Geometry: see drawing. Coordinates: mm, zero at the bounding-box minimum. A direction names the side the tool comes from. Round coordinates to 2 decimals unless told otherwise and drop trailing zeros. Loops run counter-clockwise (first coordinate to the right, second up) from the corner with the lowest first, then second, coordinate; pieces in that order, holes last.
(1) Material intervals for probe 1 along Y at (x, z) = (38, 1.5); probe 2 along X at (y, z) = (9, 1.25); probe 3 along Z at (x, y) = (33.5, 70.5), sorted ascending.
(2) Set-up query: the marked faces 1, 2 and 3. Return all of +Z, -Z, +X, -X, +Y, -Y with unobstructed straight access to the full face (end or side cutting, diameter ignored); none if empty.
(3) Section A-A, the plane x = 22.5. Return the cut outline in (y, z), plus the area to 3 significant figures.
(4) Section C-C, the plane z = 8. Return the cut outline in (x, y), plus the area to 3 significant figures.
(5) First-contact query: pin 1 Ø7 at (y, z) = (4.5, 3.5) entering from +X; pin 2 Ø1.9 at (x, y) = (45, 44) entering from +Z; pin 3 Ø5 at (x, z) = (39, 10) entering from +Y; pin 4 Ø6 at (x, y) = (11, 51) entering from -Z. Flat tips, straight axial feed; report the tip coordinate or a pass-through.
(6) Section B-B, the plane y = 36.5. Return the cut outline in (x, z), plus the area to 3 significant figures.
(7) Section D-D, the plane z = 3.75. Return the cut outline in (x, y), plus the area to 3 significant figures.
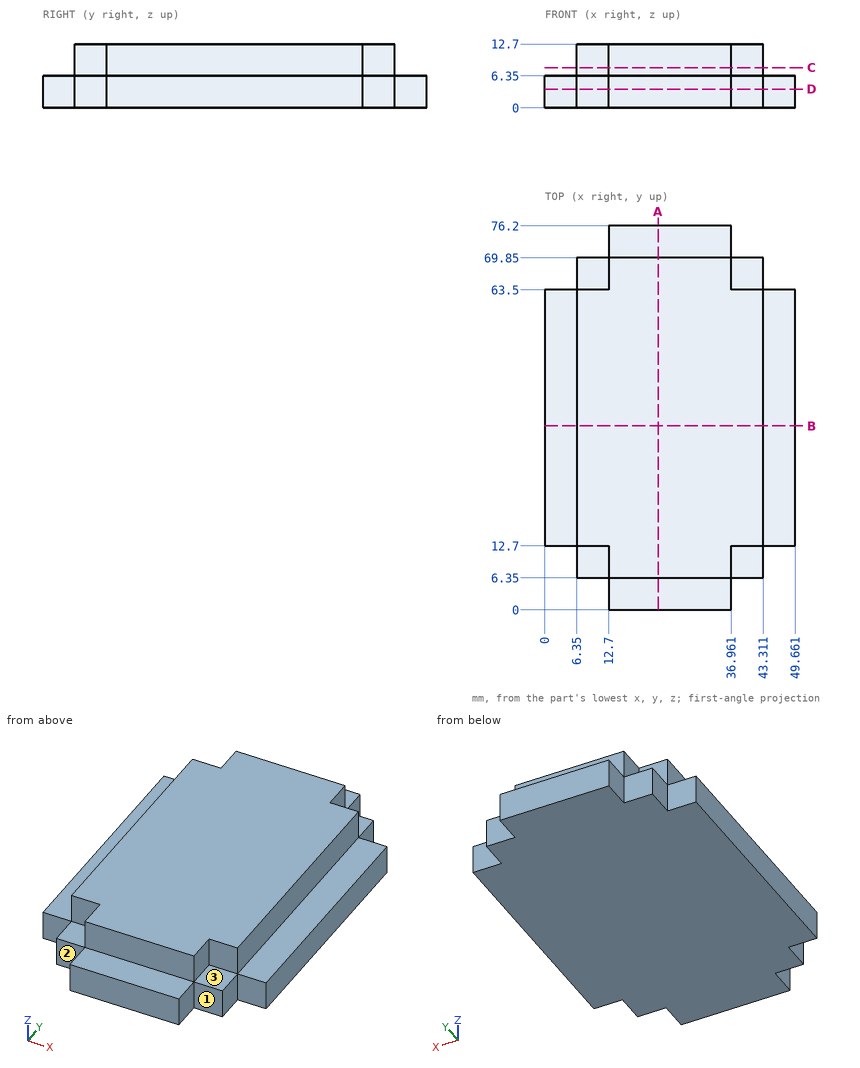
Output values:
1. probe 1: y = 6.35 to 69.85
1. probe 2: x = 6.35 to 43.31
1. probe 3: z = 0 to 6.35
2. face 1: +Z, -Z, +X, -Y
2. face 2: +Z, -Z, -X, -Y
2. face 3: +Z, +X, -Y
3. outline: (0, 0) - (76.2, 0) - (76.2, 6.35) - (69.85, 6.35) - (69.85, 12.7) - (6.35, 12.7) - (6.35, 6.35) - (0, 6.35) - close
3. area: 887 mm2
4. outline: (6.35, 12.7) - (12.7, 12.7) - (12.7, 6.35) - (36.96, 6.35) - (36.96, 12.7) - (43.31, 12.7) - (43.31, 63.5) - (36.96, 63.5) - (36.96, 69.85) - (12.7, 69.85) - (12.7, 63.5) - (6.35, 63.5) - close
4. area: 2,190 mm2
5. pin 1: stops at x = 43.31
5. pin 2: stops at z = 6.35
5. pin 3: stops at y = 69.85
5. pin 4: stops at z = 0
6. outline: (0, 0) - (49.66, 0) - (49.66, 6.35) - (43.31, 6.35) - (43.31, 12.7) - (6.35, 12.7) - (6.35, 6.35) - (0, 6.35) - close
6. area: 550 mm2
7. outline: (0, 12.7) - (6.35, 12.7) - (6.35, 6.35) - (12.7, 6.35) - (12.7, 0) - (36.96, 0) - (36.96, 6.35) - (43.31, 6.35) - (43.31, 12.7) - (49.66, 12.7) - (49.66, 63.5) - (43.31, 63.5) - (43.31, 69.85) - (36.96, 69.85) - (36.96, 76.2) - (12.7, 76.2) - (12.7, 69.85) - (6.35, 69.85) - (6.35, 63.5) - (0, 63.5) - close
7. area: 3,300 mm2
